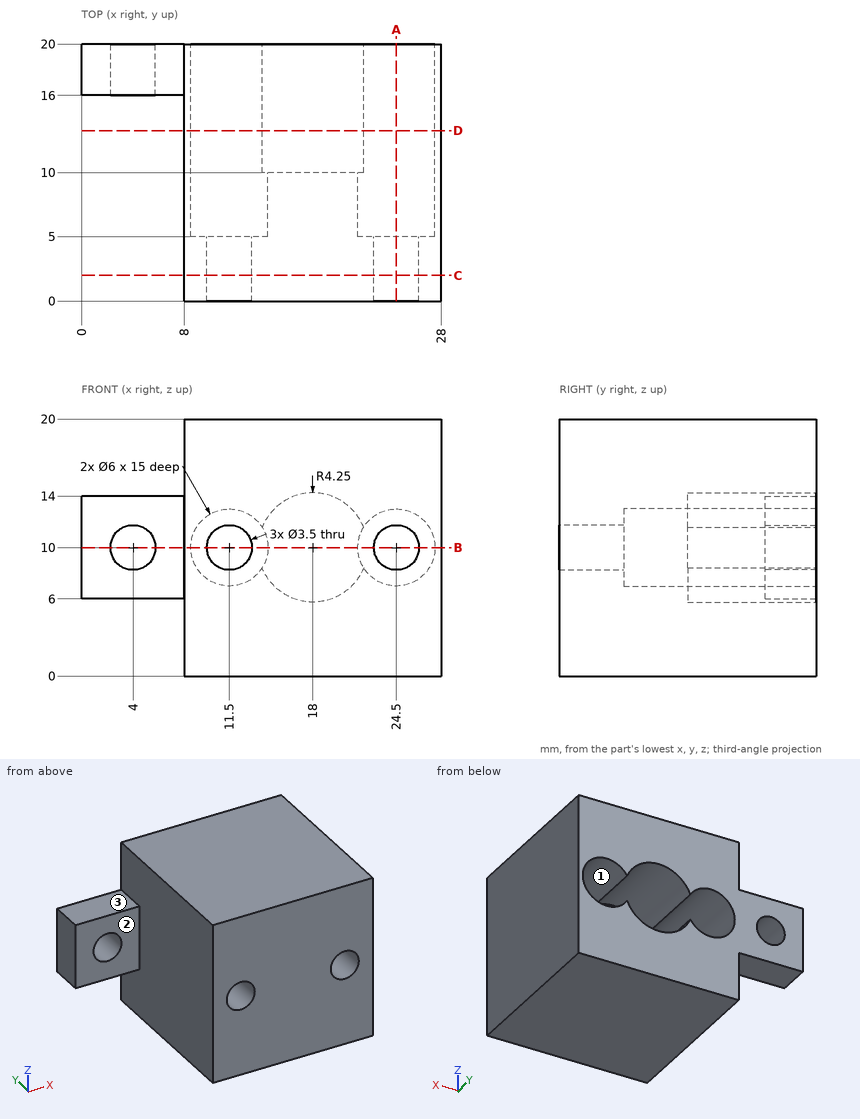
Geometry: see drawing. Coordinates: mm, zero at the bounding-box minimum. A direction names the side the tool comes from. Coordinates: 2 decimals unless noted, no trailing zeros. Loops run counter-clockwise (first coordinate to the right, second up) from the corner with the lowest first, then second, coordinate; pieces in that order, holes last. Notation, with made-up numbers: (81, 8) - (107, 8) arc R25 cw to (107, 29) - close; hole circle Ø3 at (-29.75, 78.5). An arc over 180 degrees is marked (long way). Answer as CSV lines item,"result".
1. Section C-C (y = 2). Return loops of the section in (x, z), then the cut area to 3 significant figures.
Established:
outline,"(8, 0) - (28, 0) - (28, 20) - (8, 20) - close; hole circle Ø3.5 at (11.5, 10); hole circle Ø3.5 at (24.5, 10)"
area,"381 mm2"
2. Ray query, line 1 (X direction, y = 1.5, z = 10); line 2 (X direction, y = 9.5, z = 10); line 3 (Z direction, x = 18, y = 16). Return the intervals inside material, ascending.
Established:
line 1,"x = 8 to 9.75, 13.25 to 22.75, 26.25 to 28"
line 2,"x = 8 to 8.5, 14.5 to 21.5, 27.5 to 28"
line 3,"z = 0 to 5.75, 14.25 to 20"
3. Section B-B (z = 10). Return loops of the section in (x, y).
Established:
outline,"(0, 16) - (2.25, 16) - (2.25, 20) - (0, 20) - close; (5.75, 16) - (8, 16) - (8, 0) - (9.75, 0) - (9.75, 5) - (8.5, 5) - (8.5, 20) - (5.75, 20) - close; (13.25, 0) - (22.75, 0) - (22.75, 5) - (21.5, 5) - (21.5, 10) - (14.5, 10) - (14.5, 5) - (13.25, 5) - close; (26.25, 0) - (28, 0) - (28, 20) - (27.5, 20) - (27.5, 5) - (26.25, 5) - close"
4. Contact query for flat-ended pins moving along their axis: pin 1 (4 mm diameter, centred on y = 8.5, z = 17.5, fed in from -X); pin 2 (6.5 mm diameter, centred on x = 2.5, z = 9, fed in from -Y); pin 3 (3 mm diameter, centred on x = 24.5, z = 10, fed in from +Y); pin 4 (2.5 mm diameter, centred on x = 20, z = 9.5, fed in from +Y). Output: stop coordinate, or through.
Established:
pin 1,"stops at x = 8"
pin 2,"stops at y = 16"
pin 3,"passes through"
pin 4,"stops at y = 10"
5. Section D-D (y = 13.25). Return loops of the section in (x, z), then the cut area to 3 significant figures.
Established:
outline,"(8, 0) - (28, 0) - (28, 20) - (8, 20) - close; hole (14.05, 8.42) arc R4.25 ccw to (21.95, 8.42) arc R3 ccw (long way) to (21.95, 11.58) arc R4.25 ccw to (14.05, 11.58) arc R3 ccw (long way) to start"
area,"290 mm2"
6. Reachability of the marked faces 1, 2 and 3 from +Z, -Z, +X, -X, +Y, -Y: full face, straight path, thin tool, end or side. Return the list, or none.
Established:
face 1,"+Y"
face 2,"+Z, -Z, -X, -Y"
face 3,"+Z, -X, +Y, -Y"
7. Section A-A (x = 24.5). Return loops of the section in (y, z), then the cut area to 4 significant figures.
Established:
outline,"(0, 0) - (20, 0) - (20, 7) - (5, 7) - (5, 8.25) - (0, 8.25) - close; (0, 11.75) - (5, 11.75) - (5, 13) - (20, 13) - (20, 20) - (0, 20) - close"
area,"292.5 mm2"
